Autodesk Inventor part; units mm, degrees
ref_plane "YZ Plane" through (0, 0, 0) normal (1, 0, 0) x (0, 1, 0)
ref_plane "XZ Plane" through (0, 0, 0) normal (0, 1, 0) x (-1, 0, 0)
ref_plane "XY Plane" through (0, 0, 0) normal (0, 0, 1) x (1, 0, 0)
sketch "スケッチ1" plane through (0, 0, 0) normal (0, 0, 1) x (1, 0, 0)
  line L0 (0, 4.5) -> (0, -4.5)
  line L1 (0, -4.5) -> (5.1962, -4.5)
  line L2 (5.1962, -4.5) -> (5.1962, 4.5)
  line L3 (5.1962, 4.5) -> (0, 4.5)
  point P0 (0, 0)
  point P1 (0, 0)
  dimension "d0" = 9
  dimension "d1" = 5.1962
revolve "回転1" add sketch "スケッチ1" angle 360 about axis through (0, 4.5, 0) along (0, -1, 0)
sketch "スケッチ2" plane through (0, 4.5, 0) normal (0, 1, 0) x (1, 0, 0)
  line L0 (3.4641, 0) -> (1.7321, -3)
  line L1 (1.7321, -3) -> (-1.7321, -3)
  line L2 (-1.7321, -3) -> (-3.4641, 0)
  line L3 (-3.4641, 0) -> (-1.7321, 3)
  line L4 (-1.7321, 3) -> (1.7321, 3)
  line L5 (1.7321, 3) -> (3.4641, 0)
  circle A0 centre (0, 0) radius 7.5191
  point P0 (0, 0)
  dimension "d3" = 6
extrude "押し出し1" cut sketch "スケッチ2" against normal through all
hole "穴1" at (0, 4.5, 0) direction (0, -1, 0) diameter 2.459 end through all
properties part number "ASU-309-6" material "アルミニウム 2014-T4"
Work out the finished part from the listing and answer in its coordinate system (mm). Round coordinates to 2 decimals unless told otherwise and drop trailing zeros. Loops run counter-clockwise (first coordinate to the right, second up) from the corner with the lowest first, then second, coordinate; pieces in that order, holes last. Notation, with made-up numbers: (3.25, 58.25) -> (31.25, 58.25) arc R9 ccw to (31.25, 65.25) -> close; hole circle Ø9 at (26.25, -2.5). An arc over 180 degrees is marked (long way). Write each question's results on one line, items separated by ' | '. Start each with the question number.
1. Section A-A (y = -0.5) is taken. Determine the outline of the cut face in (x, z).
2. Section B-B (x = 0) is taken. Determine the outline of the cut face in (y, z).
3. For a pull along Z with two mould halves and no side action, classify faces 1 (the face through (0, 0, -3)), 2 (the face through (0.748, -0.063, -0.976)), 3 (the face through (0, 0, 3)) as +Z half, -Z half, draft (parallel to the pull), parting line (faces both ways), or undercut.
4. Section C-C (z = 0.5) is taken. Determine the outline of the cut face in (x, y).
5. Section D-D (z = 2.75) is taken. Determine the outline of the cut face in (x, y), plus the area to 3 significant figures.
6. Find the intervals of material crossed by probe 1 along Z at (x, y) = (0, -1); probe 2 along X at (y, z) = (-1.75, -0.75); probe 3 along Z at (x, y) = (-2.5, 0), in increasing order. Write a range as from..to.
Evaluation:
1) outline: (-3.46, 0) -> (-1.73, -3) -> (1.73, -3) -> (3.46, 0) -> (1.73, 3) -> (-1.73, 3) -> close; hole circle Ø2.46 at (0, 0)
2) outline: (-4.5, -3) -> (4.5, -3) -> (4.5, -1.23) -> (-4.5, -1.23) -> close; (-4.5, 1.23) -> (4.5, 1.23) -> (4.5, 3) -> (-4.5, 3) -> close
3) face 1: -Z half | face 2: undercut | face 3: +Z half
4) outline: (-3.18, -4.5) -> (-1.12, -4.5) -> (-1.12, 4.5) -> (-3.18, 4.5) -> close; (1.12, -4.5) -> (3.18, -4.5) -> (3.18, 4.5) -> (1.12, 4.5) -> close
5) outline: (-1.88, -4.5) -> (1.88, -4.5) -> (1.88, 4.5) -> (-1.88, 4.5) -> close | area: 33.8 mm2
6) probe 1: z = -3..-1.23, 1.23..3 | probe 2: x = -3.03..-0.97, 0.97..3.03 | probe 3: z = -1.67..1.67
